Verification items for the finished model (mm, model axes). A direction names the side the tool comes from. Round coordinates to 2 decimals unless told otherwise and drop trailing zeros. Order: outer loops, then holes, each group sorted by start corner. A loop starts at its lowest first (then second) coordinate and runs counter-clockwise, first axis right, second up. Notation, with made-up numbers: (14, -32) -> (49, -32) arc R31 ccw to (49, 1) -> close; hole circle Ø5 at (25.5, -34.75). An arc over 180 degrees is marked (long way). Put each result on its own line as item: value.
from build123d import *

# Parameters (mm, degrees)
F0_W     = 203.2
F0_H     = 25.4
F1_DEPTH = 25.4
F3_R     = 9.525
F4_DEPTH = 190.5
F5_R     = 9.525
F6_DEPTH = 12.7
F2_R     = 7.14375
F7_DEPTH = 19.05


with BuildPart() as f1:
    # F0 (on Front) → F1 (new body)
    with BuildSketch(Plane.XZ):
        Rectangle(F0_W, F0_H)
    extrude(amount=F1_DEPTH)

    # F3 (on face) → F4 (cut)
    with BuildSketch(Plane.YZ.offset(101.6)):
        with Locations((-12.7, 0)):
            Circle(F3_R)
    extrude(amount=-F4_DEPTH, mode=Mode.SUBTRACT)

    # F5 (on face) → F6 (join)
    with BuildSketch(Plane.YZ.offset(101.6)):
        with Locations((-12.7, 0)):
            Circle(F5_R)
    extrude(amount=-F6_DEPTH)

    # F2 (on face) → F7 (cut)
    with BuildSketch(Plane.XZ.offset(25.4)):
        with Locations((-76.2, 0)):
            Circle(F2_R)
        with Locations((-25.4, 0)):
            Circle(F2_R)
        with Locations((25.4, 0)):
            Circle(F2_R)
        with Locations((76.2, 0)):
            Circle(F2_R)
    extrude(amount=-F7_DEPTH, mode=Mode.SUBTRACT)


solid = f1.part
Item 1: Section check A-A on z = -2. Record the boundary of the cut face in (x, y).
Check sheet entries:
outline: (-101.6, -25.4) -> (-83.06, -25.4) -> (-83.06, -22.01) -> (-88.9, -22.01) -> (-88.9, -3.39) -> (88.9, -3.39) -> (88.9, -22.01) -> (83.06, -22.01) -> (83.06, -25.4) -> (101.6, -25.4) -> (101.6, 0) -> (-101.6, 0) -> close; (-69.34, -25.4) -> (-32.26, -25.4) -> (-32.26, -22.01) -> (-69.34, -22.01) -> close; (-18.54, -25.4) -> (18.54, -25.4) -> (18.54, -22.01) -> (-18.54, -22.01) -> close; (32.26, -25.4) -> (69.34, -25.4) -> (69.34, -22.01) -> (32.26, -22.01) -> close
Item 2: Release check for a two-part mould opening along X. For faces 4 (the cylindrical face through (82.799, -22.956, -2.736)), 5 (the cylindrical face through (1.245, -3.615, 2.861)), 6 (the flat face through (-101.6, -13, 0)), 7 (the flat face through (-1, -13, -12.7)) record: +X half, -X half, draft (parallel to the pull), parting line (faces both ways), or undercut.
Check sheet entries:
face 4: undercut
face 5: undercut
face 6: -X half
face 7: draft
Item 3: Tool access check on faces 1 (the cylindrical face through (32.214, -22.956, 2.146)), 2 (the flat face through (101.6, -13, 0)), 3 (the flat face through (-88.9, -13, 0)). Record the directions out of +Z, -Z, +X, -X, +Y, -Y that give a thin tool (end or side, any length) a straight path to the whole face; none if there is none.
Check sheet entries:
face 1: -Y
face 2: +Z, -Z, +X, +Y, -Y
face 3: none
Item 4: Material ranges on L1, parallel to X at y = -23, z = 0; L2, parallel to X at y = -14.75, z = 2; L3, parallel to Z at x = 76.2, y = -21, recorded low to high. Write a range as [from, to].
Check sheet entries:
L1: x = [-101.6, -83.34], [-69.06, -32.54], [-18.26, 18.26], [32.54, 69.06], [83.34, 101.6]
L2: x = [-101.6, -88.9], [88.9, 101.6]
L3: z = [-12.7, -7.14], [7.14, 12.7]
Item 5: Gauge pin test, flat ends, axial feed: pin 1 Ø13 at (x, z) = (-76.2, 0) entering from -Y; pin 2 Ø11.5 at (x, z) = (-25.4, 0) entering from -Y; pin 3 Ø3 at (x, z) = (-54, -7.5) entering from +Y. Record the tip position at first contact, or that the pin passes through.
Check sheet entries:
pin 1: stops at y = -5.74
pin 2: stops at y = -5.11
pin 3: stops at y = 0
Item 6: Section check B-B on y = -12.7. Record the boundary of the cut face in (x, z) (3 decimals), then the cut area to 3 significant figures.
Check sheet entries:
outline: (-101.6, -12.7) -> (101.6, -12.7) -> (101.6, 12.7) -> (-101.6, 12.7) -> close; hole (-88.9, -9.525) -> (88.9, -9.525) -> (88.9, 9.525) -> (-88.9, 9.525) -> close
area: 1,770 mm^2
Item 7: Section check C-C on x = -11. Record the boundary of the cut face in (y, z) (3 decimals).
Check sheet entries:
outline: (-25.4, -12.7) -> (0, -12.7) -> (0, 12.7) -> (-25.4, 12.7) -> close; hole circle Ø19.05 at (-12.7, 0)
